from build123d import *

# Parameters (mm, degrees)
SKETCH1_W            = 115
SKETCH1_H            = 61.82
BOSS_EXTRUDE1_DEPTH  = 3
CUT_EXTRUDE1_DEPTH   = 3
SKETCH3_W            = 61.82
SKETCH3_H            = 30
BOSS_EXTRUDE2_DEPTH  = 3
SKETCH4_W            = 10
SKETCH4_H            = 3.45
BOSS_EXTRUDE3_DEPTH  = 50
SKETCH5_W            = 6
SKETCH5_H            = 2
SKETCH5_W_2          = 2
SKETCH5_H_2          = 6
BOSS_EXTRUDE12_DEPTH = 5
SKETCH8_W            = 10.631694969
SKETCH8_H            = 1.375866407
SKETCH8_H_2          = 1.500945172
CUT_EXTRUDE2_DEPTH   = 5


with BuildPart() as part:
    # Sketch1 → Boss-Extrude1 (new body)
    with BuildSketch(Plane(origin=(0, 0, 0), x_dir=(1, 0, 0), z_dir=(0, 1, 0))):
        Rectangle(SKETCH1_W, SKETCH1_H)
    extrude(amount=BOSS_EXTRUDE1_DEPTH)

    # Sketch2 → Cut-Extrude1 (cut)
    with BuildSketch(Plane(origin=(0, 3, 0), x_dir=(1, 0, 0), z_dir=(0, 1, 0))):
        with BuildLine():
            Line((-57.5, -10.91), (-57.5, -15.029841252))
            ThreePointArc((-57.5, -15.029841252), (-54.586832313, -13.823167687), (-53.380158748, -10.91))
            Line((-53.380158748, -10.91), (-53.380158748, 10.91))
            ThreePointArc((-53.380158748, 10.91), (-54.586832313, 13.823167687), (-57.5, 15.029841252))
            Line((-57.5, 15.029841252), (-57.5, 10.91))
            Line((-57.5, 10.91), (-57.5, -10.91))
        make_face()
    extrude(amount=-CUT_EXTRUDE1_DEPTH, mode=Mode.SUBTRACT)

    # Sketch3 → Boss-Extrude2 (add)
    with BuildSketch(Plane(origin=(57.5, 0, 0), x_dir=(0, 0, -1), z_dir=(1, 0, 0))):
        with Locations((0, -12)):
            Rectangle(SKETCH3_W, SKETCH3_H)
    extrude(amount=BOSS_EXTRUDE2_DEPTH)

    # Sketch4 → Boss-Extrude3 (add)
    with BuildSketch(Plane.ZY.offset(-57.5)):
        with Locations((25.91, -4.725)):
            Rectangle(SKETCH4_W, SKETCH4_H)
    boss_extrude3 = extrude(amount=BOSS_EXTRUDE3_DEPTH)

    # Mirror1: Boss-Extrude3 across plane
    add(boss_extrude3.mirror(Plane.XY))

    # Sketch5 → Boss-Extrude12 (add)
    with BuildSketch(Plane.XZ):
        with Locations((46, -14.25)):
            Rectangle(SKETCH5_W, SKETCH5_H)
        with Locations((3, -14.25)):
            Rectangle(SKETCH5_W, SKETCH5_H)
        with Locations((-1, 10.25)):
            Rectangle(SKETCH5_W_2, SKETCH5_H_2)
        with Locations((50, 10.25)):
            Rectangle(SKETCH5_W_2, SKETCH5_H_2)
    extrude(amount=BOSS_EXTRUDE12_DEPTH)

    # Sketch8 → Cut-Extrude2 (cut)
    with BuildSketch(Plane.XZ):
        with Locations((28.01669804, 17.698645154)):
            Rectangle(SKETCH8_W, SKETCH8_H)
        with Locations((28.01669804, -18.261499593)):
            Rectangle(SKETCH8_W, SKETCH8_H_2)
    extrude(amount=-CUT_EXTRUDE2_DEPTH, mode=Mode.SUBTRACT)


solid = part.part
Design review of the part built by this model. Coordinates are the model's own, in mm. A direction names the side the tool comes from. Round coordinates to 2 decimals unless told otherwise and drop trailing zeros. Loops run counter-clockwise (first coordinate to the right, second up) from the corner with the lowest first, then second, coordinate; pieces in that order, holes last. Notation, with made-up numbers: M 44.25,77.25 L 61.25,77.25 A29 ccw 61.25,105.25 Z; hole C 40.25,58.25 d1. An arc over 180 degrees is marked long. Answer as a JSON object with one key per item and string values.
Item 1: We need section C-C on x = 1.5. Give the boundary of the cut face in (y, z), and give its area (3 significant figures).
Answer sheet:
{"outline": "M -5,-15.25 L 0,-15.25 L 0,-30.91 L 3,-30.91 L 3,30.91 L 0,30.91 L 0,-13.25 L -5,-13.25 Z", "area": "195 mm^2"}
Item 2: Wall thickness on L1, parallel to Y at x = 46.5, z = 25; L2, parallel to Y at x = 44, z = -20.5; L3, parallel to X at y = -25.5, z = 15: over which ranges is each line inside the solid? List them lowest first. Write a range as from..to.
Answer sheet:
{"L1": "y = -6.45..-3, 0..3", "L2": "y = 0..3", "L3": "x = 57.5..60.5"}
Item 3: We need section D-D on y = -21.5. Give the boundary of the cut face in (x, z), and give its area (3 significant figures).
Answer sheet:
{"outline": "M 57.5,-30.91 L 60.5,-30.91 L 60.5,30.91 L 57.5,30.91 Z", "area": "185 mm^2"}
Item 4: We need section B-B on z = -23. Give the boundary of the cut face in (x, y), and give its area (4 significant figures).
Answer sheet:
{"outline": "M -57.5,0 L 57.5,0 L 57.5,-3 L 7.5,-3 L 7.5,-6.45 L 57.5,-6.45 L 57.5,-27 L 60.5,-27 L 60.5,3 L -57.5,3 Z", "area": "607.5 mm^2"}
Item 5: The part is to be moulded in two halves that separate along X. For faces 1 (the flat face through (46, -2, -15.25)), 2 (the flat face through (-53.38, 2, 0)), 3 (the flat face through (51, -2, 10)), say which applies: pulls with the +X half, pulls with the -X half, needs draft (parallel to the pull), parting line crosses it, or undercut.
Answer sheet:
{"face 1": "needs draft", "face 2": "pulls with the -X half", "face 3": "undercut"}
Item 6: Machinability: for faces 4 (the flat face through (-2, -2, 10)), 5 (the flat face through (3, -2, -13.25)), 6 (the flat face through (3, -2, -15.25)), which of the approach directions +Z, -Z, +X, -X, +Y, -Y give a long, thin tool a straight path to every point of the face, cutting with its end or side? Answer none if there is none.
Answer sheet:
{"face 4": "+Z, -Z, -X, -Y", "face 5": "+Z, -X, -Y", "face 6": "-Z, -X, -Y"}
Item 7: Clearance check with flat-ended pins moving along their axes: P1, Ø4, axis at y = -4, z = -27, coming from the -X side; P2, Ø1, axis at x = -1, y = -1.5, coming from the -Z side; P3, Ø3, axis at x = -11.5, z = -5.5, coming from the -Y side; P4, Ø12, axis at x = 18, y = -2, coming from the +Z side. State where each tip first meets the part, or that it passes through.
Answer sheet:
{"P1": "stops at x = 7.5", "P2": "stops at z = 7.25", "P3": "stops at y = 0", "P4": "stops at z = 30.91"}
Item 8: We need section A-A on x = 17. Give the boundary of the cut face in (y, z).
Answer sheet:
{"outline": "M -6.45,-30.91 L -3,-30.91 L -3,-20.91 L -6.45,-20.91 Z; M -6.45,20.91 L -3,20.91 L -3,30.91 L -6.45,30.91 Z; M 0,-30.91 L 3,-30.91 L 3,30.91 L 0,30.91 Z"}
